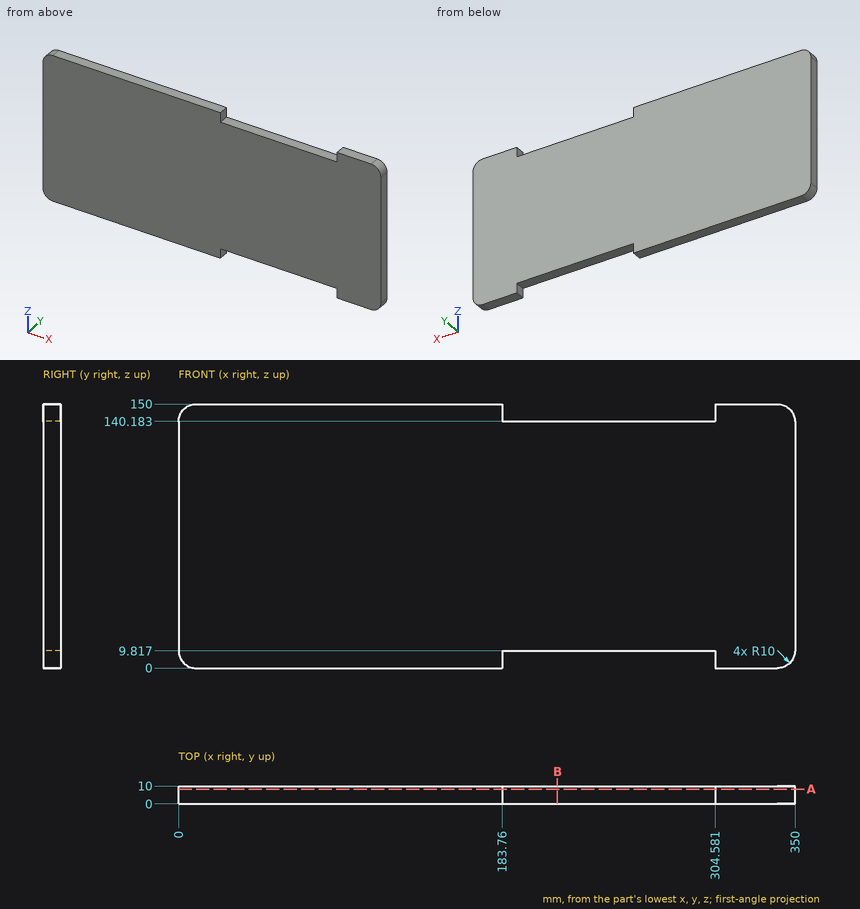
Study the drawing (mm; zero at the part's minimum x, y, z) and answer. Coordinates: 2 decimals unless noted, no trailing zeros. Write each loop counter-clockwise with the first axis right and the second up, starting at its lowest first coordinate (ties: lowest second). Pieces come first, ordered by that corner, then holes.
Q1. Section B-B, the plane x = 215 is taken. Write down the section's boundary in (y, z), then the cut area to 3 significant figures.
Returned:
outline: (0, 9.82) - (10, 9.82) - (10, 140.18) - (0, 140.18) - close
area: 1,300 mm2
Q2. Given P1, Ø3, axis at y = 6.5, z = 2.5, coming from the +X side; P2, Ø3, axis at x = 247, y = 6.5, coming from the -Z side; P3, Ø5, axis at y = 4.5, z = 143.5, coming from the -X side, each flat-ended and moving along its own axis, determine where each tip first touches the part or whether it passes through.
Returned:
P1: stops at x = 348
P2: stops at z = 9.82
P3: stops at x = 0.05
Q3. Section A-A, the plane y = 8.25 is taken. Write down the section's boundary in (x, z), then the cut area to 3 significant figures.
Returned:
outline: (0, 10) arc R10 ccw to (10, 0) - (183.76, 0) - (183.76, 9.82) - (304.58, 9.82) - (304.58, 0) - (340, 0) arc R10 ccw to (350, 10) - (350, 140) arc R10 ccw to (340, 150) - (304.58, 150) - (304.58, 140.18) - (183.76, 140.18) - (183.76, 150) - (10, 150) arc R10 ccw to (0, 140) - close
area: 50,000 mm2
Q4. Find the intervals of material crossed by line 1 along Z through (x, y) = (192, 8.5); line 2 along X through (y, z) = (9.25, 142), in increasing order.
Returned:
line 1: z = 9.82 to 140.18
line 2: x = 0.2 to 183.76, 304.58 to 349.8
